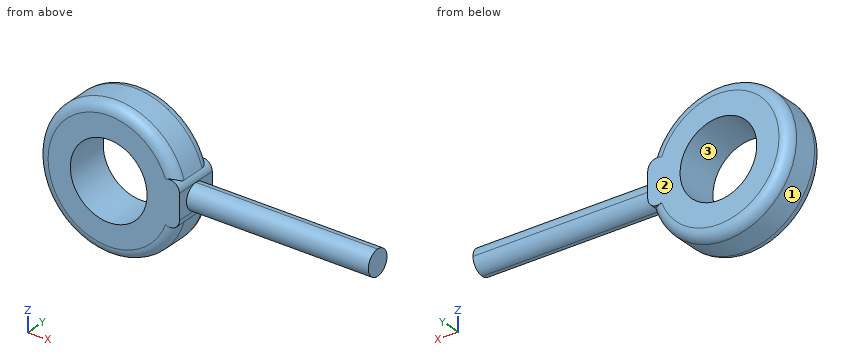
```python
from build123d import *

# Parameters (mm, degrees)
F0_R     = 4.826
F1_DEPTH = 5.588
F3_DEPTH = 22.86
F4_R     = 1.27
F5_R     = 1.27


# Not quite as in the source:
# - a feature names something its author has since deleted; it is built from what else it names


with BuildPart() as f1:
    # F0 (on Front) → F1 (new body)
    with BuildSketch(Plane.XZ):
        with BuildLine():
            Line((-22.86, -1.5875), (-22.86, 1.5875))
            ThreePointArc((-22.86, 1.5875), (-22.9466228701, 2.0329296457), (-23.1938651263, 2.4134324153))
            ThreePointArc((-23.1938651263, 2.4134324153), (-40.64, 0), (-23.1938651263, -2.4134324153))
            ThreePointArc((-23.1938651263, -2.4134324153), (-22.9466228701, -2.0329296457), (-22.86, -1.5875))
        make_face()
        with Locations((-31.75, 0)):
            Circle(F0_R, mode=Mode.SUBTRACT)
        Polygon((0, -1.5875), (0, 0), (0, 1.5875), (-22.86, 1.5875), (-22.86, -1.5875), align=None)
    extrude(amount=F1_DEPTH)

    # F2 (on face) → F3 (cut, through all)
    with BuildSketch(Plane.YZ):
        with BuildLine():
            ThreePointArc((-2.794, -1.5875), (-4.3815, 0), (-2.794, 1.5875))
            Line((-2.794, 1.5875), (-5.588, 1.5875))
            Line((-5.588, 1.5875), (-5.588, -1.5875))
            Line((-5.588, -1.5875), (-2.794, -1.5875))
        make_face()
        with BuildLine():
            ThreePointArc((-2.794, 1.5875), (-1.6714679849, 1.1225320151), (-1.2065, 0))
            ThreePointArc((-1.2065, 0), (-1.6714679849, -1.1225320151), (-2.794, -1.5875))
            Line((-2.794, -1.5875), (0, -1.5875))
            Line((0, -1.5875), (0, 1.5875))
            Line((0, 1.5875), (-2.794, 1.5875))
        make_face()
    extrude(amount=-F3_DEPTH, mode=Mode.SUBTRACT)

    # F4
    f4_edges = [f1.edges().sort_by_distance(p)[0] for p in [
        (-40.64, 0, 0),
    ]]
    fillet(f4_edges, radius=F4_R)

    # F5
    f5_edges = [f1.edges().sort_by_distance(p)[0] for p in [
        (-40.64, -5.588, 0),
    ]]
    fillet(f5_edges, radius=F5_R)


solid = f1.part
```
Geometry: final body of the model. Coordinates: model frame, mm. Face numbers are marked on the shaded views. Give positions to 0.01 mm unless a question says otherwise; leave off trailing zeros. Write each loop counter-clockwise with the first axis right and the second up, starting at its lowest first coordinate (ties: lowest second). Pieces come first, ordered by that corner, then holes.
1. Section query C-C, the plane y = -5.15. Return loops of the section in (x, z), then the cut area to 3 significant figures.
2. Section query A-A, the plane y = -1.9. Return loops of the section in (x, z).
3. Pin query (flat end, axial travel): P1, Ø0.8, axis at y = -4.5, z = 0.5, coming from the +X side; P2, Ø3, axis at x = -6.5, y = -1.5, coming from the -Z side; P3, Ø1, axis at y = -1.5, z = 2.5, coming from the -X side. Return the tip coordinate at first contact, or that it passes through.
4. Line query: probe 1 along Z at (x, y) = (-31.75, -3.55); probe 2 along X at (y, z) = (-4.85, -0.25); probe 3 along X at (y, z) = (-4.75, 1). Output: solid intervals per line, ascending.
5. Draft query along Z for the marked faces 1, 2 and 3. Return one class per face: released by +Z, released by -Z, zero draft, split by the parting line, or undercut.
6. Section query B-B, the plane x = -16.5. Return loops of the section in (y, z) (1 decimal).
Computed:
1. outline: (-23.6, -2.69) arc R1.19 ccw to (-22.86, -1.59) - (-22.86, 1.59) arc R1.19 ccw to (-23.6, 2.69) arc R8.58 ccw (long way) to start; hole circle Ø9.65 at (-31.75, 0)
1. area: 160 mm2
2. outline: (-23.19, -2.41) arc R1.19 ccw to (-22.86, -1.59) - (-22.86, -1.31) - (0, -1.31) - (0, 1.31) - (-22.86, 1.31) - (-22.86, 1.59) arc R1.19 ccw to (-23.19, 2.41) arc R8.89 ccw (long way) to start; hole circle Ø9.65 at (-31.75, 0)
3. P1: stops at x = 0
3. P2: stops at z = -1.59
3. P3: stops at x = -40.41
4. probe 1: z = -8.89 to -4.83, 4.83 to 8.89
4. probe 2: x = -40.52 to -36.57, -26.93 to -22.86
4. probe 3: x = -40.51 to -36.47, -27.03 to -22.86
5. face 1: split by the parting line
5. face 2: zero draft
5. face 3: undercut
6. outline: circle Ø3.2 at (-2.8, 0)
